Source: CAD feature listing. Evaluate the final solid. Frame: model axes, mm. A direction names the side the tool comes from. Give positions to 0.01 mm unless a question says otherwise; leave off trailing zeros. Loops run counter-clockwise (first coordinate to the right, second up) from the corner with the lowest first, then second, coordinate; pieces in that order, holes last. Notation, with made-up numbers: M -11.5,72 L 7.5,72 A15 ccw 7.5,79 Z; hole C 23,23.25 d10. An arc over 180 degrees is marked long. Put each result on its own line as item: value. Start each with the question number.
```python
from build123d import *

# Parameters (mm, degrees)
SKETCH_1_W          = 50
SKETCH_1_H          = 35.5
EXTRUDE_1_DEPTH     = 10
SKETCH_2_R          = 11.25
CUT_EXTRUDE_1_DEPTH = 33.25
SKETCH_3_R          = 1.65
CUT_EXTRUDE_2_DEPTH = 33.25
SKETCH_4_W          = 25
SKETCH_4_H          = 19.5
EXTRUDE_2_DEPTH     = 10
SKETCH_5_R          = 1.25
CUT_EXTRUDE_3_DEPTH = 10
SKETCH_7_W          = 25
SKETCH_7_H          = 10
EXTRUDE_4_DEPTH     = 11.1
SKETCH_8_W          = 2.5
SKETCH_8_H          = 10
CUT_EXTRUDE_4_DEPTH = 59.586026491
SKETCH_9_W          = 5.5
SKETCH_9_H          = 10
CUT_EXTRUDE_5_DEPTH = 5.5
SKETCH_10_W         = 10
SKETCH_10_H         = 30.6
EXTRUDE_5_DEPTH     = 3
SKETCH_11_R         = 2.75
CUT_EXTRUDE_6_DEPTH = 62.166351044
SKETCH_13_R         = 1.6
CUT_EXTRUDE_8_DEPTH = 62.166351044


with BuildPart() as part:
    # 草图1 → 凸台-拉伸1 (new body)
    with BuildSketch(Plane.XY):
        Rectangle(SKETCH_1_W, SKETCH_1_H)
    extrude(amount=EXTRUDE_1_DEPTH)

    # 草图2 → 切除-拉伸1 (cut, through all)
    with BuildSketch(Plane.XY.offset(10)):
        with Locations((0, -2.75)):
            Circle(SKETCH_2_R)
    extrude(amount=-CUT_EXTRUDE_1_DEPTH, mode=Mode.SUBTRACT)

    # 草图3 → 切除-拉伸2 (cut, through all)
    with BuildSketch(Plane.XY.offset(10)):
        with Locations((-16, -2.75)):
            Circle(SKETCH_3_R)
        with Locations((-11.313708499, 8.563708499)):
            Circle(SKETCH_3_R)
        with Locations((11.313708499, 8.563708499)):
            Circle(SKETCH_3_R)
        with Locations((16, -2.75)):
            Circle(SKETCH_3_R)
        with Locations((11.313708499, -14.063708499)):
            Circle(SKETCH_3_R)
        with Locations((-11.313708499, -14.063708499)):
            Circle(SKETCH_3_R)
    extrude(amount=-CUT_EXTRUDE_2_DEPTH, mode=Mode.SUBTRACT)

    # 草图4 → 凸台-拉伸2 (add)
    with BuildSketch(Plane.XY.offset(10)):
        with Locations((-37.5, 8)):
            Rectangle(SKETCH_4_W, SKETCH_4_H)
    extrude(amount=-EXTRUDE_2_DEPTH)

    # 草图5 → 切除-拉伸3 (cut)
    with BuildSketch(Plane(origin=(0, 0, 0), x_dir=(-1, 0, 0), z_dir=(0, 0, -1))):
        with Locations((42, 1.25)):
            Circle(SKETCH_5_R)
        with Locations((32, 1.25)):
            Circle(SKETCH_5_R)
    extrude(amount=-CUT_EXTRUDE_3_DEPTH, mode=Mode.SUBTRACT)

    # 草图7 → 凸台-拉伸4 (add)
    with BuildSketch(Plane(origin=(0, 17.75, 0), x_dir=(1, 0, 0), z_dir=(0, 1, 0))):
        with Locations((-37.5, -5)):
            Rectangle(SKETCH_7_W, SKETCH_7_H)
    extrude(amount=EXTRUDE_4_DEPTH)

    # 草图8 → 切除-拉伸4 (cut, through all)
    with BuildSketch(Plane(origin=(0, 0, 0), x_dir=(-1, 0, 0), z_dir=(0, 0, -1))):
        with Locations((45.75, 23.85)):
            Rectangle(SKETCH_8_W, SKETCH_8_H)
    extrude(amount=-CUT_EXTRUDE_4_DEPTH, mode=Mode.SUBTRACT)

    # 草图9 → 切除-拉伸5 (cut)
    with BuildSketch(Plane(origin=(0, 0, 0), x_dir=(-1, 0, 0), z_dir=(0, 0, -1))):
        with Locations((45.75, 23.85)):
            Rectangle(SKETCH_9_W, SKETCH_9_H)
    extrude(amount=-CUT_EXTRUDE_5_DEPTH, mode=Mode.SUBTRACT)

    # 草图10 → 凸台-拉伸5 (add)
    with BuildSketch(Plane.ZY.offset(50)):
        with Locations((5, 13.55)):
            Rectangle(SKETCH_10_W, SKETCH_10_H)
    extrude(amount=EXTRUDE_5_DEPTH)

    # 草图11 → 切除-拉伸6 (cut, through all)
    with BuildSketch(Plane(origin=(0, 0, 0), x_dir=(-1, 0, 0), z_dir=(0, 0, -1))):
        with Locations((45.75, 18.85)):
            Circle(SKETCH_11_R)
    extrude(amount=-CUT_EXTRUDE_6_DEPTH, mode=Mode.SUBTRACT)

    # 草图13 → 切除-拉伸8 (cut, through all)
    with BuildSketch(Plane.XY.offset(10)):
        with Locations((-50, 15.85)):
            Circle(SKETCH_13_R)
        with Locations((-40, 15.85)):
            Circle(SKETCH_13_R)
    extrude(amount=-CUT_EXTRUDE_8_DEPTH, mode=Mode.SUBTRACT)


solid = part.part
```
1. Ray query, line 1 (Y direction, x = 16, z = 7.25); line 2 (X direction, y = 9.5, z = 5.25); line 3 (X direction, y = 7.5, z = 7). Return the intervals inside material, ascending.
2. Contact query for flat-ended pins moving along their axis: pin 1 (5 mm diameter, centred on y = 22, z = 3, fed in from +X); pin 2 (1.2 mm diameter, centred on x = -44, y = 23.5, fed in from -Z). Output: stop coordinate, or through.
3. Pull-direction query (Y, two-part tool) for faces 1 (the face through (-48.52, 15.24, 5.07)), 2 (the face through (0, -17.75, 5)), 3 (the face through (-48.5, 24, 3)), 4 (the face through (0, 17.75, 5)); classes: released by +Y, released by -Y, zero draft, split by the parting line, or undercut.
4. Section B-B, the plane x = 0. Output: boundary loops of the cut face in (y, z), plus the area to 3 significant figures.
5. Section C-C, the plane x = -50. Output: boundary loops of the cut face in (y, z).
6. Section D-D, the plane z = 6.5. State how many separate pieces and enclosed holes the cut face has, plus the area to 3 significant figures.
7. Section A-A, the plane y = -2.75. Output: boundary loops of the cut face in (x, z).
8. Set-up query: faces 5 (the face through (-41, 0.5, 4.9)), 6 (the face through (-25, 23, 5)), 7 (the face through (-39, -1.75, 5)), 8 (the face through (-48, 25, 5.5)), 9 (the face through (-13, 5, 10)). Return all of +Z, -Z, +X, -X, +Y, -Y with unobstructed straight access to the full face (end or side cutting, diameter ignored); none if empty.
Results found:
1. line 1: -17.75 to -4.4, -1.1 to 17.75
1. line 2: -53 to -12.67, -9.96 to 9.96, 12.67 to 25
1. line 3: -53 to -12.58, -10.05 to -4.64, 4.64 to 10.05, 12.58 to 25
2. pin 1: x = -25
2. pin 2: z = 5.5
3. face 1: undercut
3. face 2: released by -Y
3. face 3: zero draft
3. face 4: released by +Y
4. outline: M -17.75,0 L -14,0 L -14,10 L -17.75,10 Z; M 8.5,0 L 17.75,0 L 17.75,10 L 8.5,10 Z
4. area: 130 mm²
5. outline: M -1.75,0 L 14.25,0 L 14.25,10 L -1.75,10 Z; M 17.45,0 L 28.85,0 L 28.85,10 L 17.45,10 Z
6. separate pieces: 1
6. enclosed holes: 11
6. area: 2,110 mm²
7. outline: M -25,0 L -17.65,0 L -17.65,10 L -25,10 Z; M -14.35,0 L -11.25,0 L -11.25,10 L -14.35,10 Z; M 11.25,0 L 14.35,0 L 14.35,10 L 11.25,10 Z; M 17.65,0 L 25,0 L 25,10 L 17.65,10 Z
8. face 5: +Z, -Z
8. face 6: +Z, -Z, +X, +Y
8. face 7: +Z, -Z, -X, -Y
8. face 8: -Z, +Y
8. face 9: +Z, +X, -X, +Y, -Y
